from build123d import *

# Parameters (mm, degrees)
SKETCH_2_W               = 720
SKETCH_2_H               = 720
EXTRUDE_2_DEPTH          = 405
CUT_EXTRUDE_1_DEPTH      = 270
CUT_EXTRUDE_2_DEPTH      = 651.557453266
CUT_EXTRUDE_2_DEPTH_BACK = 651.557453266
SKETCH_3_R               = 10


with BuildPart() as part:
    # 草图2 → 凸台-拉伸2 (new, symmetric)
    with BuildSketch(Plane(origin=(0, 0, 0), x_dir=(1, 0, 0), z_dir=(0, 1, 0))):
        Rectangle(SKETCH_2_W, SKETCH_2_H)
    extrude(amount=EXTRUDE_2_DEPTH, both=True)

    # 草图1 → 切除-拉伸1 (cut, symmetric)
    with BuildSketch(Plane(origin=(0, 0, 0), x_dir=(1, 0, 0), z_dir=(0, 1, 0))):
        with BuildLine():
            Line((330, 0), (330, -360))
            Line((330, -360), (-330, -360))
            Line((-330, -360), (-330, 0))
            ThreePointArc((-330, 0), (0, 330), (330, 0))
        make_face()
    extrude(amount=CUT_EXTRUDE_1_DEPTH, both=True, mode=Mode.SUBTRACT)

    # 草图3 → 切除-拉伸2 (cut, two sides: drawn at the far end of the back side and taken through both)
    with BuildSketch(Plane(origin=(0, 0, 0), x_dir=(1, 0, 0), z_dir=(0, 1, 0)).offset(-CUT_EXTRUDE_2_DEPTH_BACK)):
        with Locations(Location((0, 0, 0), (0, 0, 270))):
            Circle(SKETCH_3_R)
    extrude(amount=CUT_EXTRUDE_2_DEPTH + CUT_EXTRUDE_2_DEPTH_BACK, mode=Mode.SUBTRACT)


solid = part.part
Geometry check sheet. Reference: the model listing, model coordinates, mm. A direction names the side the tool comes from. Round coordinates to 2 decimals unless told otherwise and drop trailing zeros. Write each loop counter-clockwise with the first axis right and the second up, starting at its lowest first coordinate (ties: lowest second). Pieces come first, ordered by that corner, then holes.
Item 1: Section check D-D (z = -161). Record the boundary of the cut face in (x, y), plus the area to 3 significant figures.
Determined:
outline: (-360, -405) - (360, -405) - (360, 405) - (-360, 405) - close; hole (-288.06, -270) - (288.06, -270) - (288.06, 270) - (-288.06, 270) - close
area: 272,000 mm2
Item 2: Material ranges on line 1 along X through (y, z) = (-265, 49); line 2 along Y through (x, z) = (-283, 49); line 3 along X through (y, z) = (310, 0), recorded low to high.
Determined:
line 1: x = -360 to -330, 330 to 360
line 2: y = -405 to -270, 270 to 405
line 3: x = -360 to -10, 10 to 360
Item 3: Section check B-B (x = -57.5). Record the boundary of the cut face in (y, z), plus the area to 3 significant figures.
Determined:
outline: (-405, -360) - (405, -360) - (405, 360) - (270, 360) - (270, -324.95) - (-270, -324.95) - (-270, 360) - (-405, 360) - close
area: 213,000 mm2
Item 4: Section check C-C (y = -242). Record the boundary of the cut face in (x, z), plus the area to 3 significant figures.
Determined:
outline: (-360, -360) - (360, -360) - (360, 360) - (330, 360) - (330, 0) arc R330 cw to (-330, 0) - (-330, 360) - (-360, 360) - close
area: 110,000 mm2
Item 5: Section check A-A (z = 24.5). Record the boundary of the cut face in (x, y).
Determined:
outline: (-360, -405) - (360, -405) - (360, 405) - (-360, 405) - close; hole (-330, -270) - (330, -270) - (330, 270) - (-330, 270) - close
Item 6: Access from +Z, -Z, +X, -X, +Y, -Y to the whole of each face (thin tool, end or side, straight path). Record for faces 1 (the face through (330, 4, 177)), 2 (the face through (-360, 6, 5)).
Determined:
face 1: +Z
face 2: +Z, -Z, -X, +Y, -Y
Item 7: Mould release check, pull along Z, two halves, no side actions. Record for faces 3 (the face through (-5, -405, -85)), 4 (the face through (-9.76, 336.55, -2.17)), 5 (the face through (-5, 6, -360)): +Z half, -Z half, draft (parallel to the pull), parting line (faces both ways), or undercut.
Determined:
face 3: draft
face 4: undercut
face 5: -Z half
